from build123d import *

# Parameters (mm, degrees)
F1_R     = 43.0377999141
F1_R_2   = 1.5875
F2_DEPTH = 6.35
F0_R     = 5.4640621861
F3_DEPTH = 6.35


with BuildPart() as f2:
    # F1 (on Top) → F2 (new body)
    with BuildSketch(Plane.XY):
        with Locations((-13.9420051128, -8.2401288673)):
            Circle(F1_R)
        with Locations((-13.9420051128, 30.6853711327)):
            Circle(F1_R_2, mode=Mode.SUBTRACT)
    extrude(amount=F2_DEPTH)

    # F0 (on Top) → F3 (cut)
    with BuildSketch(Plane.XY):
        with Locations((-11.8682515955, 21.6185524797)):
            Circle(F0_R)
        with BuildLine():
            Line((-30.777075401, -0.5462395027), (-26.2022968359, -1.6195531011))
            ThreePointArc((-26.2022968359, -1.6195531011), (-25.2430473169, -1.4625330212), (-24.6757854404, -0.6732112182))
            Line((-24.6757854404, -0.6732112182), (-20.8609066441, 15.5869254009))
            ThreePointArc((-20.8609066441, 15.5869254009), (-21.017926724, 16.54617492), (-21.807248527, 17.1134367965))
            Line((-21.807248527, 17.1134367965), (-26.3820270921, 18.1867503949))
            ThreePointArc((-26.3820270921, 18.1867503949), (-27.3412766111, 18.029730315), (-27.9085384876, 17.240408512))
            Line((-27.9085384876, 17.240408512), (-31.7234172839, 0.9802718929))
            ThreePointArc((-31.7234172839, 0.9802718929), (-31.566397204, 0.0210223738), (-30.777075401, -0.5462395027))
        make_face()
        with BuildLine():
            Line((-16.4839141071, -12.11008057), (-9.9019641905, -39.0468699637))
            ThreePointArc((-9.9019641905, -39.0468699637), (-5.3848753387, -41.6411280094), (-3.0142599717, -37.0027609169))
            Line((-3.0142599717, -37.0027609169), (-10.9454579651, -3.5498633515))
            add(Edge.make_bspline(
                [(-10.9454579651, -3.5498633515), (-11.1008232007, -3.029964733), (-11.4148845809, -1.9182603696), (-11.5758558718, 0.0611210161), (-10.7270246335, 1.1480561674), (-10.4112150148, 1.642682706)],
                knots=[0, 0, 0, 0, 0.3212196894, 0.6614579708, 1, 1, 1, 1], degree=3))
            add(Edge.make_bspline(
                [(-10.4112150148, 1.642682706), (-10.3324407758, 1.1105596752), (-10.3150494323, 0.00946776), (-10.1153730649, -1.3596205713), (-9.2167931712, -1.9914203558), (-8.5628340021, -2.2260230035)],
                knots=[0, 0, 0, 0, 0.3448186812, 0.6485748194, 1, 1, 1, 1], degree=3))
            Line((-8.5628340021, -2.2260230035), (0.6940379972, -4.768232815))
            ThreePointArc((0.6940379972, -4.768232815), (3.6159208044, -3.1049103484), (1.9518018235, -0.1834811119))
            Line((1.9518018235, -0.1834811119), (-5.7092916164, 1.9159893078))
            Line((-5.7092916164, 1.9159893078), (-8.030090481, 11.0155502334))
            ThreePointArc((-8.030090481, 11.0155502334), (-13.2287628949, 15.0547445073), (-18.4274353087, 11.0155502334))
            Line((-18.4274353087, 11.0155502334), (-29.8210121691, -37.0027609169))
            ThreePointArc((-29.8210121691, -37.0027609169), (-27.4845954692, -41.6285261383), (-22.9910892352, -39.0468699637))
            Line((-22.9910892352, -39.0468699637), (-16.4839141071, -12.11008057))
        make_face()
        with BuildLine():
            Line((8.6775599048, 8.5290158167), (-0.2638578007, -40.083643049))
            ThreePointArc((-0.2638578007, -40.083643049), (0.6472478334, -41.5319603397), (2.0893774927, -40.6110920012))
            Line((2.0893774927, -40.6110920012), (10.9268212691, 8.164270781))
            ThreePointArc((10.9268212691, 8.164270781), (9.9879647619, 9.4922508691), (8.6775599048, 8.5290158167))
        make_face()
    extrude(amount=F3_DEPTH, mode=Mode.SUBTRACT)


solid = f2.part
Could you check a few things on this model? Use its own coordinates, in mm. Coordinates: 2 decimals unless noted, no trailing zeros. Write each loop counter-clockwise with the first axis right and the second up, starting at its lowest first coordinate (ties: lowest second). Pieces come first, ordered by that corner, then holes. Notation, with made-up numbers: (70.25, 67.25) - (87.25, 67.25) arc R20 cw to (87.25, 97.25) - close; hole circle Ø8 at (2.5, -38.75). An arc over 180 degrees is marked (long way). Write item = value, one per line.
1) Please list where these lines run through material, in increasing order: line 1 (X direction, y = 6.5, z = 4.25); line 2 (X direction, y = -15, z = 5.25); line 3 (X direction, y = -10, z = 1.5). Write a range as [from, to].
Result set:
line_1 = [-54.38, -30.43], [-22.99, -19.5], [-6.88, 8.3], [10.63, 26.49]
line_2 = [-56.45, -24.6], [-17.18, -15.78], [-8.23, 4.35], [6.73, 28.56]
line_3 = [-56.94, -23.41], [-9.42, 5.27], [7.64, 29.06]
2) Suppose I cut it at D-D on x = 22.5. Please give me the cut outline in (y, z).
Result set:
outline = (-31.14, 0) - (14.66, 0) - (14.66, 6.35) - (-31.14, 6.35) - close
3) Will these pins go through, and if not, where does the flat tip stop? pin 1 Ø5 at (x, y) = (-13.94, 30.69) entering from +Z; pin 2 Ø1 at (y, z) = (-36.5, 4) entering from -X.
Result set:
pin_1 = 6.35
pin_2 = -46.83
4) Suppose I cut it at C-C on z = 1.5. State how many separate pieces and enclosed holes the cut face has, plus the area to 3 significant figures.
Result set:
separate_pieces = 1
enclosed_holes = 5
area = 4,660 mm2
5) Suppose I cut it at A-A on y = 4. Please give me the cut outline in (x, z), plus the area to 3 significant figures.
Result set:
outline = (-55.2, 0) - (-31.01, 0) - (-31.01, 6.35) - (-55.2, 6.35) - close; (-23.58, 0) - (-20.09, 0) - (-20.09, 6.35) - (-23.58, 6.35) - close; (-6.24, 0) - (7.84, 0) - (7.84, 6.35) - (-6.24, 6.35) - close; (10.17, 0) - (27.32, 0) - (27.32, 6.35) - (10.17, 6.35) - close
area = 374 mm2
6) We'd pull the mould along X, two halves only. Please class faces 1 (the cylindrical face through (27.108, 4.687, 3.131)), 2 (the cylindrical face through (3.6, -3.16, 3.13)), 3 (the flat face through (-5, -8, 6.35)), 4 (the flat face through (-4, -3.48, 3.13)): +X half, -X half, draft (parallel to the pull), parting line (faces both ways), or undercut.
Result set:
face_1 = parting line
face_2 = undercut
face_3 = draft
face_4 = undercut
7) Suppose I cut it at B-B on x = -4. Please give me the cut outline in (y, z), plus the area to 3 significant figures.
Result set:
outline = (-50.11, 0) - (-40.86, 0) - (-40.86, 6.35) - (-50.11, 6.35) - close; (-32.85, 0) - (-3.48, 0) - (-3.48, 6.35) - (-32.85, 6.35) - close; (1.45, 0) - (33.63, 0) - (33.63, 6.35) - (1.45, 6.35) - close
area = 450 mm2
